```python
from build123d import *

# Parameters (mm, degrees)
PAD038_DEPTH         = 37.5
SKETCH074_R          = 7
POCKET033_DEPTH      = 50
SKETCH075_R          = 11.2
POCKET034_DEPTH      = 7
CHAMFER033_SIZE      = 1
SKETCH085_W          = 18
SKETCH085_H          = 18
POCKET043_DEPTH      = 19
CHAMFER036_SIZE      = 2
SKETCH086_R          = 3.2
POCKET044_DEPTH      = 6.001
POCKET044_DEPTH_BACK = 24.001
CHAMFER037_SIZE      = 1
CHAMFER038_SIZE      = 1
CHAMFER039_SIZE      = 0.8


with BuildPart() as part:
    # Sketch073 → Pad038 (new body, symmetric)
    with BuildSketch(Plane.XZ):
        with BuildLine():
            ThreePointArc((15, 0), (0, 15), (-15, 0))
            Line((-15, 0), (-15, -31))
            Line((-15, -31), (15, -31))
            Line((15, -31), (15, 0))
        make_face()
    extrude(amount=PAD038_DEPTH, both=True)

    # Sketch074 → Pocket033 (cut, symmetric)
    with BuildSketch(Plane.XZ):
        Circle(SKETCH074_R)
    extrude(amount=POCKET033_DEPTH, both=True, mode=Mode.SUBTRACT)

    # Sketch075 (on Face5 of Pocket033) → Pocket034 (cut)
    with BuildSketch(Plane.XZ.offset(37.5)):
        Circle(SKETCH075_R)
    pocket034 = extrude(amount=-POCKET034_DEPTH, mode=Mode.SUBTRACT)

    # Mirrored002: Pocket034 across XZ
    add(pocket034.mirror(Plane.XZ), mode=Mode.SUBTRACT)

    # Chamfer033
    chamfer033_edges = [part.edges().sort_by_distance(p)[0] for p in [
        (-11.2, 37.5, 0),
        (-7, 30.5, 0),
        (-11.2, -37.5, 0),
        (-7, -30.5, 0),
    ]]
    chamfer(chamfer033_edges, length=CHAMFER033_SIZE)

    # Sketch085 (on Face6 of Chamfer033) → Pocket043 (cut)
    with BuildSketch(Plane(origin=(0, 0, -31), x_dir=(1, 0, 0), z_dir=(0, 0, -1))):
        with Locations((0, 16.5)):
            Rectangle(SKETCH085_W, SKETCH085_H)
    extrude(amount=-POCKET043_DEPTH, mode=Mode.SUBTRACT)

    # Chamfer036
    chamfer036_edges = [part.edges().sort_by_distance(p)[0] for p in [
        (9, -25.5, -21.5),
        (9, -7.5, -21.5),
        (-9, -7.5, -21.5),
        (-9, -25.5, -21.5),
    ]]
    chamfer(chamfer036_edges, length=CHAMFER036_SIZE)

    # Sketch086 (on Face5 of Chamfer036) → Pocket044 (cut, two sides)
    with BuildSketch(Plane(origin=(9, 0, 0), x_dir=(0, 0, -1), z_dir=(-1, 0, 0))) as pocket044_sk:
        with Locations((21.5, 16.5)):
            Circle(SKETCH086_R)
    extrude(amount=-POCKET044_DEPTH, mode=Mode.SUBTRACT)
    extrude(pocket044_sk.sketch, amount=POCKET044_DEPTH_BACK, mode=Mode.SUBTRACT)

    # Chamfer037
    chamfer037_edges = [part.edges().sort_by_distance(p)[0] for p in [
        (15, 37.5, -15.5),
        (15, -37.5, -15.5),
    ]]
    chamfer(chamfer037_edges, length=CHAMFER037_SIZE)

    # Chamfer038
    chamfer038_edges = [part.edges().sort_by_distance(p)[0] for p in [
        (9, -16.5, -18.3),
        (-15, -16.5, -18.3),
        (-9, -16.5, -18.3),
        (15, -16.5, -18.3),
    ]]
    chamfer(chamfer038_edges, length=CHAMFER038_SIZE)

    # Chamfer039
    chamfer039_edges = [part.edges().sort_by_distance(p)[0] for p in [
        (-15, 0, -31),
        (-14.5, 37, -31),
        (-14.5, -37, -31),
        (0, 37.5, -31),
        (0, -37.5, -31),
        (14.5, 37, -31),
        (14.5, -37, -31),
        (15, 0, -31),
        (0, -25.5, -31),
        (8, -24.5, -31),
        (-8, -24.5, -31),
        (9, -16.5, -31),
        (-9, -16.5, -31),
        (8, -8.5, -31),
        (-8, -8.5, -31),
        (0, -7.5, -31),
    ]]
    chamfer(chamfer039_edges, length=CHAMFER039_SIZE)


solid = part.part
```
Input: part model. Units: mm. Frame: model coordinates. A direction names the side the tool comes from. Round coordinates to 2 decimals unless told otherwise and drop trailing zeros. Loops run counter-clockwise (first coordinate to the right, second up) from the corner with the lowest first, then second, coordinate; pieces in that order, holes last. Notation, with made-up numbers: (14.5, -3.5) -> (70.5, -3.5) arc R21 ccw to (70.5, 19.5) -> close; hole circle Ø11 at (-12.5, 71). An arc over 180 degrees is marked (long way). Write each question's results on one line, items separated by ' | '.
1. Section C-C (y = -16.5). State how many separate pieces and enclosed holes the cut face has, and give its area (3 significant figures).
Geometry results:
separate pieces: 3 | enclosed holes: 1 | area: 705 mm2
2. Set-up query: faces 1 (the face through (9, -16, -17)), 2 (the face through (12, -16.6, -18.3)), 3 (the face through (-8, 30.5, 3)). Return all of +Z, -Z, +X, -X, +Y, -Y with unobstructed straight access to the full face (end or side cutting, diameter ignored); none if empty.
Geometry results:
face 1: -Z | face 2: +X, -X | face 3: +Y
3. Section D-D (z = -14). Return loops of the section in (x, y).
Geometry results:
outline: (-15, -36.5) -> (-14, -37.5) -> (14, -37.5) -> (15, -36.5) -> (15, 36.5) -> (14, 37.5) -> (-14, 37.5) -> (-15, 36.5) -> close; hole (-9, -23.5) -> (-7, -25.5) -> (7, -25.5) -> (9, -23.5) -> (9, -9.5) -> (7, -7.5) -> (-7, -7.5) -> (-9, -9.5) -> close
4. First-contact query: P1, Ø7.5, axis at y = -16.5, z = -21.5, coming from the +X side; P2, Ø8.5, axis at x = 0, z = 0, coming from the +Y side; P3, Ø4, axis at x = 0, z = 7.5, coming from the +Y side; P4, Ø3, axis at x = -1.5, z = -6, coming from the +Y side. Flat tips, straight axial feed; report the tip coordinate or a pass-through.
Geometry results:
P1: x = 14.55 | P2: through | P3: y = 30.5 | P4: y = 30.18
5. Ray query, line 1 (Y direction, x = 2.5, z = -28); line 2 (Z direction, x = 0, y = -34.15); line 3 (Y direction, x = 12.65, z = -21.5). Return the intervals inside material, ascending. Write a range as from..to.
Geometry results:
line 1: -37.5..-25.5, -7.5..37.5 | line 2: -31..-11.2, 11.2..15 | line 3: -37.5..-19.7, -13.3..37.5
6. Mould query, pull axis Y, two halves, no side actions, for faces 4 (the face through (-9, -16, -17)), 5 (the face through (0, -37.5, -13)), 6 (the face through (6.466, -0.413, -2.681)). Classes: +Y half, -Y half, draft (parallel to the pull), parting line (faces both ways), or undercut.
Geometry results:
face 4: undercut | face 5: -Y half | face 6: draft
